Source: CAD feature listing. Evaluate the final solid. Frame: model axes, mm. A direction names the side the tool comes from. Round coordinates to 2 decimals unless told otherwise and drop trailing zeros. Write each loop counter-clockwise with the first axis right and the second up, starting at its lowest first coordinate (ties: lowest second). Pieces come first, ordered by that corner, then holes. Notation, with made-up numbers: (71.5, 37.5) -> (102.5, 37.5) arc R28 ccw to (102.5, 61.5) -> close; hole circle Ø5 at (61.5, 78.25). An arc over 180 degrees is marked (long way). Put each result on its own line as item: value.
```python
from build123d import *

# Parameters (mm, degrees)
SKETCH3_R               = 4.826
CUT_EXTRUDE1_DEPTH      = 25.4
CUT_EXTRUDE2_DEPTH      = 56.71060233
CUT_EXTRUDE2_DEPTH_BACK = 56.71060233
SKETCH4_R               = 1.5
SKETCH5_R               = 1.5
CUT_EXTRUDE3_DEPTH      = 6.35
CIRPATTERN1_COUNT       = 8
SKETCH6_R               = 4.7625
BOSS_EXTRUDE1_DEPTH     = 9.525
CHAMFER1_SIZE           = 0.635


with BuildPart() as part:
    # 草图1 → 旋转1 (revolve)
    with BuildSketch(Plane.XY, mode=Mode.PRIVATE) as revolve_1_sk:
        Polygon((0, 0), (0, 30.48), (0, 49.53), (6.35, 49.53), (18.034, 30.48), (18.034, 0), align=None)
    revolve(revolve_1_sk.sketch.rotate(Axis((0, 0, 0), (0, 1, 0)), 90), axis=Axis((0, 0, 0), (0, 1, 0)))

    # Sketch3 → Cut-Extrude1 (cut)
    with BuildSketch(Plane(origin=(0, 49.53, 0), x_dir=(1, 0, 0), z_dir=(0, 1, 0))):
        with Locations(Location((0, 0, 0), (0, 0, 270))):
            Circle(SKETCH3_R)
    extrude(amount=-CUT_EXTRUDE1_DEPTH, mode=Mode.SUBTRACT)

    # Sketch4 → Cut-Extrude2 (cut, two sides: drawn at the far end of the back side and taken through both)
    with BuildSketch(Plane.XY.offset(-CUT_EXTRUDE2_DEPTH_BACK)):
        with Locations((0, 43.18)):
            Circle(SKETCH4_R)
        with Locations((0, 33.655)):
            Circle(SKETCH4_R)
    extrude(amount=CUT_EXTRUDE2_DEPTH + CUT_EXTRUDE2_DEPTH_BACK, mode=Mode.SUBTRACT)

    # Sketch5 → Cut-Extrude3 (cut)
    with BuildSketch(Plane.XZ):
        with Locations(Location((0, 9.525, 0), (0, 0, 270))):
            Circle(SKETCH5_R)
    cut_extrude3 = extrude(amount=-CUT_EXTRUDE3_DEPTH, mode=Mode.SUBTRACT)

    # CirPattern1: Cut-Extrude3 ×8 about axis
    cirpattern1_axis = Axis((0, 0, 0), (0, 1, 0))
    for i in range(1, CIRPATTERN1_COUNT):
        add(cut_extrude3.rotate(cirpattern1_axis, i * 360 / CIRPATTERN1_COUNT), mode=Mode.SUBTRACT)

    # Sketch6 → Boss-Extrude1 (add)
    with BuildSketch(Plane.XZ):
        with Locations(Location((0, 0, 0), (0, 0, 90))):
            Circle(SKETCH6_R)
    extrude(amount=BOSS_EXTRUDE1_DEPTH)

    # Chamfer1
    chamfer1_edges = [part.edges().sort_by_distance(p)[0] for p in [
        (0, -9.525, -4.7625),
    ]]
    chamfer(chamfer1_edges, length=CHAMFER1_SIZE)

    # Sketch7 → Revolve1 (revolve)
    with BuildSketch(Plane.XY, mode=Mode.PRIVATE) as revolve1_sk:
        Polygon((-5.588, 0), (-4.7625, -2.2225), (-4.7625, 0), align=None)
    revolve(revolve1_sk.sketch.rotate(Axis((0, 0, 0), (0, -1, 0)), 90), axis=Axis((0, 0, 0), (0, -1, 0)))


solid = part.part
```
Q1. Draft query along Z for faces 1 (the cylindrical face through (2.9, -5.51, -3.78)), 2 (the cylindrical face through (-0.325, 41.716, -7.191)), 3 (the flat face through (0, 6.35, -10)). Return one class per face: +Z half, -Z half, draft (parallel to the pull), parting line (faces both ways), or undercut.
Ans:
face 1: parting line
face 2: draft
face 3: undercut
Q2. Cut plane B-B on y = 43.18. Output: boundary loops of the cut face in (x, z), and give its area (3 significant figures).
Ans:
outline: (-1.5, -10.13) -> (-1.5, -4.59) arc R4.83 cw to (-1.5, 4.59) -> (-1.5, 10.13) arc R10.24 ccw to start; (1.5, -10.13) arc R10.24 ccw to (1.5, 10.13) -> (1.5, 4.59) arc R4.83 cw to (1.5, -4.59) -> close
area: 224 mm^2
Q3. Reachability of faces 4 (the flat face through (0, 24.13, 0)), 5 (the flat face through (7, 6.35, -7)), 6 (the cylindrical face through (-0.33, 32.19, -10.88)) from +Z, -Z, +X, -X, +Y, -Y: full face, straight path, thin tool, end or side. Return the list, or none.
Ans:
face 4: +Y
face 5: -Y
face 6: +Z, -Z
Q4. Material intervals for line 1 (X direction, y = 43.18, z = -7.25); line 2 (Y direction, x = 2, z = -0.5) (3 decimals); line 3 (Y direction, x = 8.5, z = -5.5), sorted ascending. Write a range as [from, to].
Ans:
line 1: x = [-7.24, -1.5], [1.5, 7.24]
line 2: y = [-9.525, 24.13]
line 3: y = [0, 43.38]
Q5. Cut plane C-C on y = 18. Output: boundary loops of the cut face in (x, z), and give its area (3 significant figures).
Ans:
outline: circle Ø36.07 at (0, 0)
area: 1,020 mm^2
Q6. Pin query (flat end, axial travel): pin 1 (3.5 mm diameter, centred on x = -0.5, z = -9.5, fed in from -Y); pin 2 (8 mm diameter, centred on x = -9, z = -14.5, fed in from +Y); pin 3 (4 mm diameter, centred on x = 0, y = 43.18, fed in from +Z). Return the tip coordinate at first contact, or that it passes through.
Ans:
pin 1: stops at y = 0
pin 2: stops at y = 38.58
pin 3: stops at z = 11.47
